Build history of the part. All positions in model axes, mm. A direction names the side the tool comes from. Coordinates: 2 decimals unless noted, no trailing zeros. Loops run counter-clockwise (first coordinate to the right, second up) from the corner with the lowest first, then second, coordinate; pieces in that order, holes last.
Item 1: Flat gauge pins, fed straight in: pin 1 (2 mm diameter, centred on x = 49, z = 2.5, fed in from -Y); pin 2 (12 mm diameter, centred on x = 21, z = 8.5, fed in from +Y); pin 3 (4.5 mm diameter, centred on y = 49.5, z = 11, fed in from -X); pin 4 (3.5 mm diameter, centred on x = 59, y = 21, fed in from -Z). Where does each tip first touch, or does it go through?
Item 2: Cut at B-B (z = 11). List the corners of the cut face in (x, y).
Item 3: 3-axis set-ups, long thin cutter, end or side, ignore diameter. For faces 1 (the face through (48, 33, 21)), 2 (the face through (55, 47, 11)), 3 (the face through (2, 40, 11)), 4 (the face through (1, 38, 11)): which of +Z, -Z, +X, -X, +Y, -Y reach the whole face in a straight line?
Item 4: Cut at A-A (x = 59). List the corners of the cut face in (y, z), and give its area (3 significant figures).
Item 5: Mould opens along Y. For faces 5 (the face through (32, 27, 0)), 6 (the face through (33, 42, 12)), 7 (the face through (27, 44, 11)), 8 (the face through (33, 12, 11)) say: released by +Y, released by -Y, zero draft, split by the parting line, or undercut.
Item 6: Drill centre lines: line 1 along Z through (x, y) = (4, 29); line 2 along Z through (x, y) = (59.5, 49.5); line 3 along Y through (x, z) = (22.5, 17). Where is each one in solid material? Low to high.
Item 7: Cut at D-D (z = 18.75). List the corners of the cut face in (x, y).
Item 8: Cut at C-C (y = 21). List the corners of the cut face in (x, z).
from build123d import *

# Parameters (mm, degrees)
BOX003_W          = 63
BOX003_H          = 30
BOX003_DEPTH      = 18
CYLINDER002_R     = 2
CYLINDER002_DEPTH = 22
BOX005_W          = 17
BOX005_H          = 17
BOX005_DEPTH      = 20
BOX004_W          = 65
BOX004_H          = 22
BOX004_DEPTH      = 18
CYLINDER001_R     = 2
CYLINDER001_DEPTH = 65
CYLINDER_R        = 2
CYLINDER_DEPTH    = 65
BOX002_W          = 55
BOX002_H          = 10
BOX002_DEPTH      = 22
BOX001_W          = 55
BOX001_H          = 10
BOX001_DEPTH      = 22
BOX_W             = 65
BOX_H             = 54
BOX_DEPTH         = 22


with BuildPart() as cavitycutout:
    # Box003 → Box003 (new body)
    with BuildSketch(Plane(origin=(2, 12, 2), x_dir=(1, 0, 0), z_dir=(0, 0, 1))):
        with Locations((31.5, 15)):
            Rectangle(BOX003_W, BOX003_H)
    extrude(amount=BOX003_DEPTH)


with BuildPart() as capturescrewhole:
    # Cylinder002 → Cylinder002 (new body)
    with BuildSketch(Plane(origin=(59, 21, 0), x_dir=(1, 0, 0), z_dir=(0, 0, 1))):
        Circle(CYLINDER002_R)
    extrude(amount=CYLINDER002_DEPTH)


with BuildPart() as cutawaynotch:
    # Box005 → Box005 (new body)
    with BuildSketch(Plane(origin=(48, 25, 2), x_dir=(1, 0, 0), z_dir=(0, 0, 1))):
        with Locations((8.5, 8.5)):
            Rectangle(BOX005_W, BOX005_H)
    extrude(amount=BOX005_DEPTH)


with BuildPart() as interiorcut:
    # Box004 → Box004 (new body)
    with BuildSketch(Plane(origin=(0, 16, 2), x_dir=(1, 0, 0), z_dir=(0, 0, 1))):
        with Locations((32.5, 11)):
            Rectangle(BOX004_W, BOX004_H)
    extrude(amount=BOX004_DEPTH)

    # Fusion003: union CavityCutOut, CaptureScrewHole, CutAwayNotch
    add(cavitycutout.part)
    add(capturescrewhole.part)
    add(cutawaynotch.part)


with BuildPart() as righthole:
    # Cylinder001 → Cylinder001 (new body)
    with BuildSketch(Plane(origin=(0, 49.5, 11), x_dir=(0, 0, -1), z_dir=(1, 0, 0))):
        Circle(CYLINDER001_R)
    extrude(amount=CYLINDER001_DEPTH)


with BuildPart() as mountingholes:
    # Cylinder → Cylinder (new body)
    with BuildSketch(Plane(origin=(0, 4.5, 11), x_dir=(0, 0, -1), z_dir=(1, 0, 0))):
        Circle(CYLINDER_R)
    extrude(amount=CYLINDER_DEPTH)

    # Fusion001: union RightHole
    add(righthole.part)


with BuildPart() as rightcut:
    # Box002 → Box002 (new body)
    with BuildSketch(Plane(origin=(0, 44, 0), x_dir=(1, 0, 0), z_dir=(0, 0, 1))):
        with Locations((27.5, 5)):
            Rectangle(BOX002_W, BOX002_H)
    extrude(amount=BOX002_DEPTH)


with BuildPart() as cutoutsandmounting:
    # Box001 → Box001 (new body)
    with BuildSketch(Plane.XY):
        with Locations((27.5, 5)):
            Rectangle(BOX001_W, BOX001_H)
    extrude(amount=BOX001_DEPTH)

    # Fusion: union RightCut
    add(rightcut.part)

    # Fusion002: union MountingHoles
    add(mountingholes.part)


with BuildPart() as ethernetmount:
    # Box → Box (new body)
    with BuildSketch(Plane.XY):
        with Locations((32.5, 27)):
            Rectangle(BOX_W, BOX_H)
    extrude(amount=BOX_DEPTH)

    # Cut: cut CutoutsAndMounting
    add(cutoutsandmounting.part, mode=Mode.SUBTRACT)

    # Cut001: cut InteriorCut
    add(interiorcut.part, mode=Mode.SUBTRACT)


solid = ethernetmount.part
Filled sheet:
1. pin 1: stops at y = 10
1. pin 2: stops at y = 44
1. pin 3: stops at x = 55
1. pin 4: passes through
2. outline: (0, 10) - (55, 10) - (55, 6.5) - (65, 6.5) - (65, 12) - (2, 12) - (2, 16) - (0, 16) - close; (0, 38) - (2, 38) - (2, 42) - (65, 42) - (65, 47.5) - (55, 47.5) - (55, 44) - (0, 44) - close; (55, 0) - (65, 0) - (65, 2.5) - (55, 2.5) - close; (55, 51.5) - (65, 51.5) - (65, 54) - (55, 54) - close
3. face 1: +Z, +X
3. face 2: +Z, -Z, -X, +Y
3. face 3: +X
3. face 4: +X, -X
4. outline: (0, 0) - (19, 0) - (19, 2) - (12, 2) - (12, 20) - (19, 20) - (19, 22) - (0, 22) - close; (23, 0) - (54, 0) - (54, 22) - (42, 22) - (42, 2) - (23, 2) - close; (23, 20) - (25, 20) - (25, 22) - (23, 22) - close; hole circle Ø4 at (4.5, 11); hole circle Ø4 at (49.5, 11)
4. area: 573 mm2
5. face 5: zero draft
5. face 6: undercut
5. face 7: released by +Y
5. face 8: undercut
6. line 1: z = 0 to 2, 20 to 22
6. line 2: z = 0 to 9, 13 to 22
6. line 3: y = 10 to 12, 42 to 44
7. outline: (0, 10) - (55, 10) - (55, 0) - (65, 0) - (65, 12) - (2, 12) - (2, 16) - (0, 16) - close; (0, 38) - (2, 38) - (2, 42) - (65, 42) - (65, 54) - (55, 54) - (55, 44) - (0, 44) - close
8. outline: (0, 0) - (57, 0) - (57, 2) - (0, 2) - close; (0, 20) - (57, 20) - (57, 22) - (0, 22) - close; (61, 0) - (65, 0) - (65, 2) - (61, 2) - close; (61, 20) - (65, 20) - (65, 22) - (61, 22) - close
